Could you check a few things on this model? Use its own coordinates, in mm. Face numbers are marked on the shaded views. Round coordinates to 2 decimals unless told otherwise and drop trailing zeros. Loops run counter-clockwise (first coordinate to the right, second up) from the corner with the lowest first, then second, coordinate; pieces in that order, holes last. Notation, with made-up numbers: (83.5, -31) -> (122.5, -31) arc R25 cw to (122.5, 0) -> close; hole circle Ø9 at (-35.5, 72). An arc over 180 degrees is marked (long way). Put each result on its own line as item: value. Start each with the question number.
1. Imagine slicing it at C-C, the plane z = 0. Please give me the cut outline in (x, y).
2. I need wall thicknesses on line 1 (X direction, y = 0.5, z = 66.5); line 2 (Z direction, x = -27, y = 3.5); line 3 (X direction, y = -4, z = 4.5). Which ranges of each line are inside material? Lowest first, please. Write a range as [from, to].
3. If we mould it in two halves opening along X, with no side actions, what happens to the marked faces 1, 2 and 3? For each: pulls with the +X half, pulls with the -X half, needs draft (parallel to the pull), parting line crosses it, or undercut.
4. Imagine slicing it at D-D, the plane y = -0.5. Please give me the cut outline in (x, z), and give its area (3 significant figures).
5. Imagine slicing it at B-B, the plane x = 0. Please give me the cut outline in (y, z).
6. Imagine slicing it at A-A, the plane z = 66.5. Please give me the cut outline in (x, y).
7. I'm going to push flat-ended pins straight in: P1, Ø6, axis at x = -23.5, y = 2, coming from the -Z side; P2, Ø3, axis at x = 20.5, y = 2.5, coming from the -Z side. Where does each tip first touch, or does it pass through?
```python
from build123d import *

# Parameters (mm, degrees)
SKETCH2_W              = 73
SKETCH2_H              = 73
SKETCH2_R              = 31.5
BOSS_EXTRUDE2_DEPTH    = 6.35
SKETCH3_W              = 73
SKETCH3_H              = 40
SKETCH3_R              = 2.5
BOTTOM_MOUNT_DEPTH     = 12.7
BOTTOM_MOUNT_FILLETS_R = 20


with BuildPart() as part:
    # Sketch2 → Boss-Extrude2 (new, symmetric)
    with BuildSketch(Plane(origin=(0, 0, 0), x_dir=(1, 0, 0), z_dir=(0, 1, 0))):
        Rectangle(SKETCH2_W, SKETCH2_H)
        with Locations(Location((0, 0, 0), (0, 0, 270))):
            Circle(SKETCH2_R, mode=Mode.SUBTRACT)
    extrude(amount=BOSS_EXTRUDE2_DEPTH, both=True)

    # Sketch3 → Bottom Mount (add, through all)
    with BuildSketch(Plane(origin=(0, 6.35, 0), x_dir=(1, 0, 0), z_dir=(0, 1, 0))):
        with Locations((0, -56.5)):
            Rectangle(SKETCH3_W, SKETCH3_H)
        with Locations(Location((-26.5, -66.5, 0), (0, 0, 270))):
            Circle(SKETCH3_R, mode=Mode.SUBTRACT)
        with Locations(Location((26.5, -66.5, 0), (0, 0, 270))):
            Circle(SKETCH3_R, mode=Mode.SUBTRACT)
    extrude(amount=-BOTTOM_MOUNT_DEPTH)

    # Bottom Mount Fillets
    bottom_mount_fillets_edges = [part.edges().sort_by_distance(p)[0] for p in [
        (-36.5, 0, -36.5),
        (36.5, 0, -36.5),
    ]]
    fillet(bottom_mount_fillets_edges, radius=BOTTOM_MOUNT_FILLETS_R)


solid = part.part
```
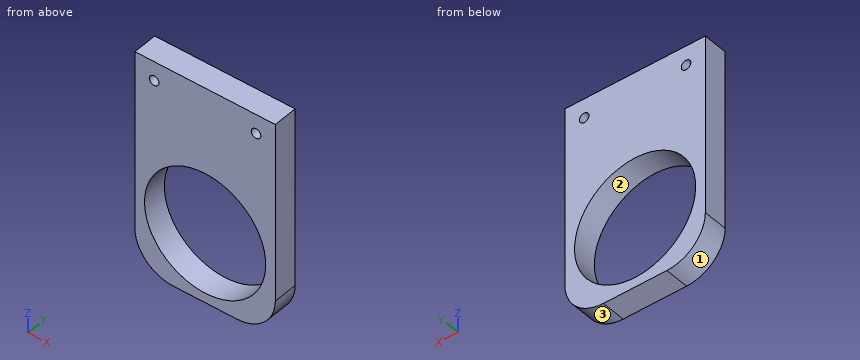
Entries:
1. outline: (-36.5, -6.35) -> (-31.5, -6.35) -> (-31.5, 6.35) -> (-36.5, 6.35) -> close; (31.5, -6.35) -> (36.5, -6.35) -> (36.5, 6.35) -> (31.5, 6.35) -> close
2. line 1: [-36.5, -29], [-24, 24], [29, 36.5]
2. line 2: [-33.52, -16.22], [16.22, 64.05], [68.95, 76.5]
2. line 3: [-36.5, -31.18], [31.18, 36.5]
3. face 1: pulls with the -X half
3. face 2: undercut
3. face 3: pulls with the +X half
4. outline: (-36.5, -16.5) arc R20 ccw to (-16.5, -36.5) -> (16.5, -36.5) arc R20 ccw to (36.5, -16.5) -> (36.5, 76.5) -> (-36.5, 76.5) -> close; hole circle Ø63 at (0, 0); hole circle Ø5 at (-26.5, 66.5); hole circle Ø5 at (26.5, 66.5)
4. area: 4,920 mm^2
5. outline: (-6.35, -36.5) -> (6.35, -36.5) -> (6.35, -31.5) -> (-6.35, -31.5) -> close; (-6.35, 31.5) -> (6.35, 31.5) -> (6.35, 76.5) -> (-6.35, 76.5) -> close
6. outline: (-36.5, -6.35) -> (-29, -6.35) -> (-29, 6.35) -> (-36.5, 6.35) -> close; (-24, -6.35) -> (24, -6.35) -> (24, 6.35) -> (-24, 6.35) -> close; (29, -6.35) -> (36.5, -6.35) -> (36.5, 6.35) -> (29, 6.35) -> close
7. P1: z = -36.1
7. P2: z = -36.34
